Read the model definition and answer for the solid it produces. Units are mm, in the model's axes. Face numbers are marked on the shaded views. A direction names the side the tool comes from. Coordinates: 2 decimals unless noted, no trailing zeros. Loops run counter-clockwise (first coordinate to the right, second up) from the corner with the lowest first, then second, coordinate; pieces in that order, holes last. Notation, with made-up numbers: (70, 39.25) -> (85, 39.25) arc R16 ccw to (85, 60.25) -> close; hole circle Ø2 at (37.5, -13.5). An arc over 180 degrees is marked (long way). Answer as a JSON object with one key per item and string values. Group by question number.
Q1. The part is cut by section C-C on y = -98. Write down the section's boundary in (x, z), and give its area (3 significant figures).
Q2. For the marked faces 1 and 2, determine the directions among +Z, -Z, +X, -X, +Y, -Y from which every point of the face is accessible in a straight line to the end or side of a thin tool.
Q3. The part is cut by section B-B on x = -19. Write down the section's boundary in (y, z), and give its area (3 significant figures).
Q4. Straight lines are drawn through the part: line 1 along Y through (x, z) = (-18, -2.25); line 2 along Z through (x, y) = (-20.5, -113); line 3 along X through (y, z) = (-106, 2.75). For each, find the intervals that lie inside material, in ascending order. Write a range as [from, to].
Q5. The part is cut by section A-A on z = 0. Write down the section's boundary in (x, y).
Q6. Each of these flat-tipped pins is pushed along its axis until it touches: P1, Ø2, axis at x = -17, y = -113.5, coming from the +Z side; P2, Ø2, axis at x = -17.5, y = -121.5, coming from the +Z side; P3, Ø5, axis at y = -127, z = 2.5, coming from the +X side. Where does it stop, or does it pass through?
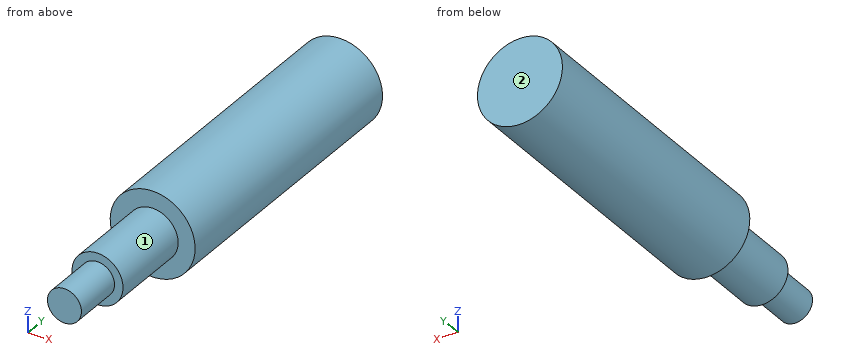
from build123d import *

# Parameters (mm, degrees)
M4_THREAD_BLANK_SKETCH_R = 2
M4_THREAD_BLANK_DEPTH    = 6
LOCATING_SPIGOT_SKETCH_R = 3
LOCATING_SPIGOT_DEPTH    = 10
GUIDE_SHOULDER_SKETCH_R  = 5
GUIDE_SHOULDER_DEPTH     = 34


with BuildPart() as part:
    # M4 Thread Blank Sketch → M4 Thread Blank (new body)
    with BuildSketch(Plane(origin=(0, -140, 0), x_dir=(1, 0, 0), z_dir=(0, 1, 0))):
        with Locations(Location((-20.291651246, 0, 0), (0, 0, 270))):
            Circle(M4_THREAD_BLANK_SKETCH_R)
    extrude(amount=M4_THREAD_BLANK_DEPTH)

    # Locating Spigot Sketch → Locating Spigot (add)
    with BuildSketch(Plane(origin=(0, -134, 0), x_dir=(1, 0, 0), z_dir=(0, 1, 0))):
        with Locations(Location((-20.291651246, 0, 0), (0, 0, 270))):
            Circle(LOCATING_SPIGOT_SKETCH_R)
    extrude(amount=LOCATING_SPIGOT_DEPTH)

    # Guide Shoulder Sketch → Guide Shoulder (add)
    with BuildSketch(Plane(origin=(0, -124, 0), x_dir=(1, 0, 0), z_dir=(0, 1, 0))):
        with Locations(Location((-20.291651246, 0, 0), (0, 0, 270))):
            Circle(GUIDE_SHOULDER_SKETCH_R)
    extrude(amount=GUIDE_SHOULDER_DEPTH)


solid = part.part
Final values:
{
 "1": {"outline": "circle Ø10 at (-20.29, 0)", "area": "78.5 mm2"},
 "2": {"face 1": "-Y", "face 2": "+Z, -Z, +X, -X, +Y"},
 "3": {"outline": "(-140, -1.53) -> (-134, -1.53) -> (-134, -2.71) -> (-124, -2.71) -> (-124, -4.83) -> (-90, -4.83) -> (-90, 4.83) -> (-124, 4.83) -> (-124, 2.71) -> (-134, 2.71) -> (-134, 1.53) -> (-140, 1.53) -> close", "area": "401 mm2"},
 "4": {"line 1": "y = [-124, -90]", "line 2": "z = [-5, 5]", "line 3": "x = [-24.47, -16.12]"},
 "5": {"outline": "(-25.29, -124) -> (-23.29, -124) -> (-23.29, -134) -> (-22.29, -134) -> (-22.29, -140) -> (-18.29, -140) -> (-18.29, -134) -> (-17.29, -134) -> (-17.29, -124) -> (-15.29, -124) -> (-15.29, -90) -> (-25.29, -90) -> close"},
 "6": {"P1": "stops at z = 4.44", "P2": "stops at z = 4.67", "P3": "stops at x = -17.29"}
}
